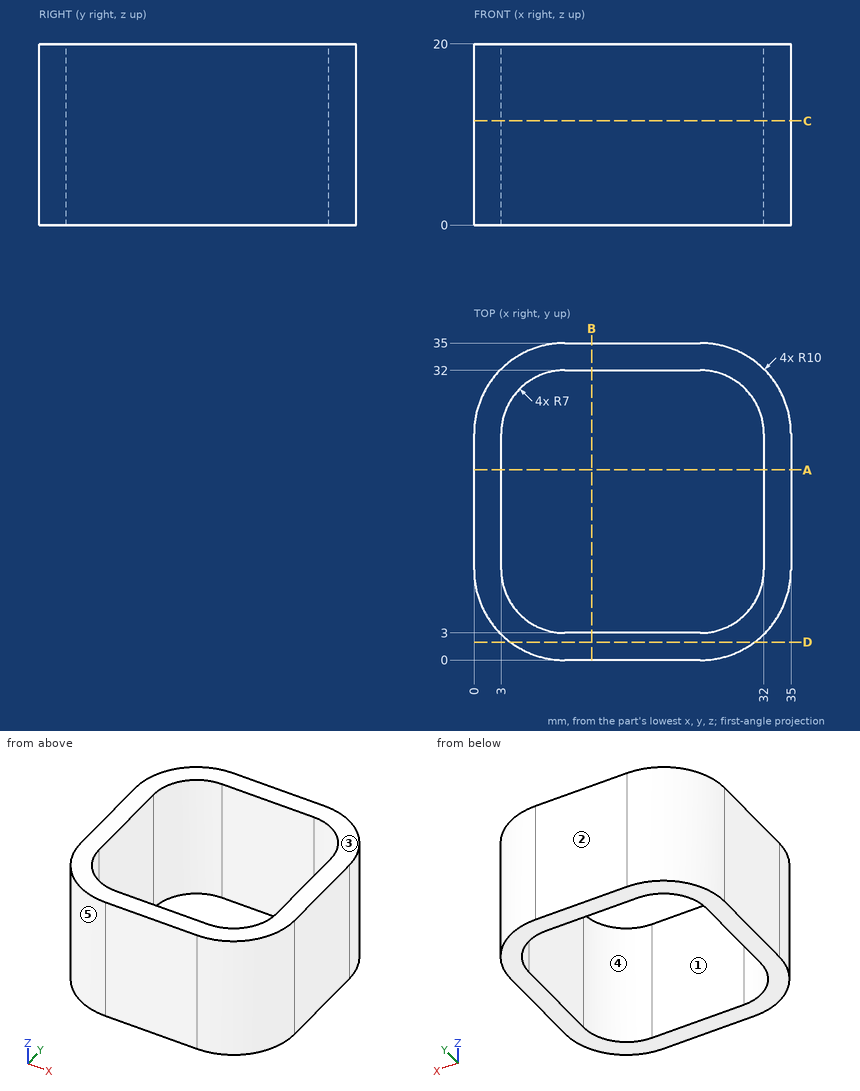
Study the drawing (mm; zero at the part's minimum x, y, z) and answer. A direction names the side the tool comes from. Give positions to 0.01 mm unless a question says otherwise; leave off trailing zeros. Order: outer loops, then holes, each group sorted by start corner. A loop starts at its lowest first (then second) coordinate and runs counter-clockwise, first axis right, second up. Notation, with made-up numbers: (6.5, 23) - (17.5, 23) arc R25 cw to (17.5, 53) - close; hole circle Ø3 at (33, 38). An arc over 180 degrees is marked (long way). Answer in a Markdown table with one row per item. Add a question column.
Q1. For a pull along X with two mould halves and no side action, classify the marked faces 3, 4 and 5 as released by +X, released by -X, zero draft, split by the parting line, or undercut.
Q2. Which of the six approach directions +Z, -Z, +X, -X, +Y, -Y give full straight-line access (tool end or side, diameter ignored) to the marked faces 1 and 2?
Q3. Given P1, Ø6, axis at y = 5, z = 14.5, coming from the +X side; P2, Ø1.5, axis at x = 30, z = 8, coming from the -Y side, each flat-ended and moving along its own axis, determine where each tip first touches the part or whether it passes through.
Q4. The part is cut by section C-C (z = 11.5). Determine the outline of the cut face in (x, y).
Q5. The part is cut by section D-D (y = 2). Determine the outline of the cut face in (x, z).
Q6. The part is cut by section A-A (y = 21). Determine the outline of the cut face in (x, z).
Q7. Find the intervals of material crossed by line 1 along X through (y, z) = (25, 12.5); line 2 along X through (y, z) = (6, 14), in increasing order. Write a range as [from, to].
Determined:
| question | item | result |
|---|---|---|
| 1 | face 3 | zero draft |
| 1 | face 4 | undercut |
| 1 | face 5 | released by -X |
| 2 | face 1 | +Z, -Z |
| 2 | face 2 | +Z, -Z, +X, -X, +Y |
| 3 | P1 | stops at x = 34.8 |
| 3 | P2 | stops at y = 0.95 |
| 4 | outline | (0, 10) arc R10 ccw to (10, 0) - (25, 0) arc R10 ccw to (35, 10) - (35, 25) arc R10 ccw to (25, 35) - (10, 35) arc R10 ccw to (0, 25) - close; hole (3, 10) arc R7 ccw to (10, 3) - (25, 3) arc R7 ccw to (32, 10) - (32, 25) arc R7 ccw to (25, 32) - (10, 32) arc R7 ccw to (3, 25) - close |
| 5 | outline | (4, 0) - (31, 0) - (31, 20) - (4, 20) - close |
| 6 | outline | (0, 0) - (3, 0) - (3, 20) - (0, 20) - close; (32, 0) - (35, 0) - (35, 20) - (32, 20) - close |
| 7 | line 1 | x = [0, 3], [32, 35] |
| 7 | line 2 | x = [0.83, 4.26], [30.74, 34.17] |
